Part model, mm, in its own coordinate system. Round coordinates to 2 decimals unless told otherwise and drop trailing zeros. Loops run counter-clockwise (first coordinate to the right, second up) from the corner with the lowest first, then second, coordinate; pieces in that order, holes last. Notation, with made-up numbers: M 3.25,52 L 53.25,52 A20 ccw 53.25,62 Z; hole C 22,89.25 d2. An arc over 180 degrees is marked long. Put each result on its own line as item: value. Start each with the question number.
```python
from build123d import *

# Parameters (mm, degrees)
EXTRUDE1_DEPTH    = 0.254
CIRPATTERN1_COUNT = 4


with BuildPart() as part:
    # Sketch2 → Extrude1 (new, symmetric)
    with BuildSketch(Plane.XY):
        with BuildLine():
            Line((-0.1524, 3.7084), (-0.1524, 3.048))
            ThreePointArc((-0.1524, 3.048), (-0.122642049, 2.976157951), (-0.0508, 2.9464))
            Line((-0.0508, 2.9464), (0.0508, 2.9464))
            ThreePointArc((0.0508, 2.9464), (0.122642049, 2.976157951), (0.1524, 3.048))
            Line((0.1524, 3.048), (0.1524, 3.7084))
            ThreePointArc((0.1524, 3.7084), (0.211915902, 3.852084098), (0.3556, 3.9116))
            Line((0.3556, 3.9116), (0.4318, 3.9116))
            ThreePointArc((0.4318, 3.9116), (0.521602561, 3.948797439), (0.5588, 4.0386))
            Line((0.5588, 4.0386), (0.5588, 4.1656))
            ThreePointArc((0.5588, 4.1656), (0.573678976, 4.201521024), (0.6096, 4.2164))
            Line((0.6096, 4.2164), (3.6576, 4.2164))
            ThreePointArc((3.6576, 4.2164), (3.837205122, 4.142005122), (3.9116, 3.9624))
            Line((3.9116, 3.9624), (3.9116, 0.762))
            Line((3.9116, 0.762), (2.0066, 0.762))
            Line((2.0066, 0.762), (2.0066, 1.905))
            ThreePointArc((2.0066, 1.905), (1.976842049, 1.976842049), (1.905, 2.0066))
            Line((1.905, 2.0066), (-0.889, 2.0066))
            Line((-0.889, 2.0066), (-0.889, 3.9116))
            Line((-0.889, 3.9116), (-0.3556, 3.9116))
            ThreePointArc((-0.3556, 3.9116), (-0.211915902, 3.852084098), (-0.1524, 3.7084))
        make_face()
    extrude1 = extrude(amount=EXTRUDE1_DEPTH, both=True)

    # CirPattern1: Extrude1 ×4 about axis
    cirpattern1_axis = Axis((0, 0, 0), (0, 0, 1))
    for i in range(1, CIRPATTERN1_COUNT):
        add(extrude1.rotate(cirpattern1_axis, i * 360 / CIRPATTERN1_COUNT))


solid = part.part
```
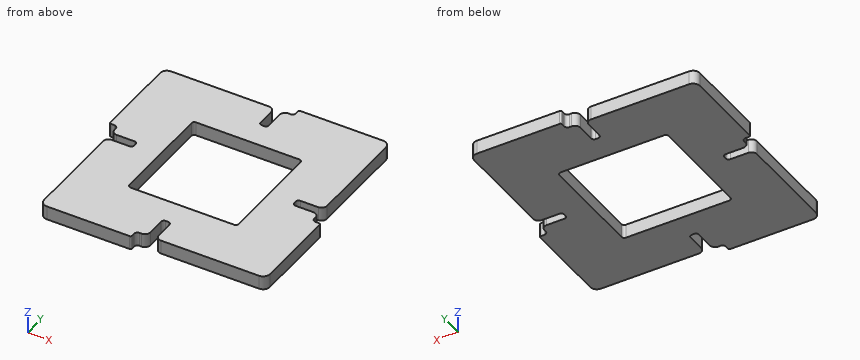
1. Cut at B-B, the plane x = 3.25. Give the cut face in (y, z).
2. Cut at A-A, the plane y = -1.75. Give the cut face in (x, z).
3. Cut at C-C, the plane y = 2.5. Give the cut face in (x, z).
4. Wall check: L1, parallel to Y at x = -1.5, z = 0.05; L2, parallel to X at y = -3.5, z = -0.05; L3, parallel to X at y = -1, z = 0. Give the ranges that are in metal, low to high.
Results list:
1. outline: M -3.91,-0.25 L -0.15,-0.25 L -0.15,0.25 L -3.91,0.25 Z; M 0.15,-0.25 L 4.22,-0.25 L 4.22,0.25 L 0.15,0.25 Z
2. outline: M -3.91,-0.25 L -2.01,-0.25 L -2.01,0.25 L -3.91,0.25 Z; M 2.01,-0.25 L 4.22,-0.25 L 4.22,0.25 L 2.01,0.25 Z
3. outline: M -4.22,-0.25 L 3.91,-0.25 L 3.91,0.25 L -4.22,0.25 Z
4. L1: y = -4.22 to -2.01, 2.01 to 3.91
4. L2: x = -3.91 to -0.15, 0.15 to 4.22
4. L3: x = -3.91 to -2.01, 2.01 to 4.22
